Build history of the part. All positions in model axes, mm. A direction names the side the tool comes from. Round coordinates to 2 decimals unless told otherwise and drop trailing zeros. Write each loop counter-clockwise with the first axis right and the second up, starting at its lowest first coordinate (ties: lowest second). Pieces come first, ordered by that corner, then holes. Notation, with made-up numbers: (12.25, -38.75) -> (21.25, -38.75) arc R23 cw to (21.25, -11.75) -> close; hole circle Ø8 at (-16.5, 4). An arc over 180 degrees is marked (long way). Answer in a Markdown table with one row per item.
```python
from build123d import *

# Parameters (mm, degrees)
F0_W          = 203.2
F0_H          = 203.2
F1_DEPTH      = 304.8
F2_W          = 127
F2_H          = 228.6
F3_DEPTH      = 25.4
F3_DEPTH_BACK = 203.2


with BuildPart() as f1:
    # F0 (on Front) → F1 (new body)
    with BuildSketch(Plane.XZ):
        Rectangle(F0_W, F0_H)
    extrude(amount=-F1_DEPTH)

    # F2 (on face) → F3 (cut, two sides)
    with BuildSketch(Plane.XY.offset(101.6)) as f3_sk:
        with Locations((0, 152.4)):
            Rectangle(F2_W, F2_H)
    extrude(amount=F3_DEPTH, mode=Mode.SUBTRACT)
    extrude(f3_sk.sketch, amount=-F3_DEPTH_BACK, mode=Mode.SUBTRACT)


solid = f1.part
```
Q1. Which spindle directions (+Z, -Z, +X, -X, +Y, -Y) get a long thin tool onto all of the face, cutting with end or side? Do faces 5 (the flat face through (-1, 38.1, 1)), 6 (the flat face through (66, 150, -101.6)). Say none if no direction does.
A:
| item | result |
|---|---|
| face 5 | +Z, -Z |
| face 6 | -Z, +X, -X, +Y, -Y |
Q2. Wall check: line 1 (Y direction, x = 23, z = -2.5); line 2 (X direction, y = 178.5, z = 87). Give the ranges that are in metal, low to high. Write a range as [from, to].
A:
| item | result |
|---|---|
| line 1 | [0, 38.1], [266.7, 304.8] |
| line 2 | [-101.6, -63.5], [63.5, 101.6] |
Q3. Saw through at A-A on x = 19. Write the cut outline in (y, z).
A:
| item | result |
|---|---|
| outline | (0, -101.6) -> (38.1, -101.6) -> (38.1, 101.6) -> (0, 101.6) -> close; (266.7, -101.6) -> (304.8, -101.6) -> (304.8, 101.6) -> (266.7, 101.6) -> close |
Q4. Saw through at C-C on z = -58.5. Write the cut outline in (x, y), plus the area to 3 significant figures.
A:
| item | result |
|---|---|
| outline | (-101.6, 0) -> (101.6, 0) -> (101.6, 304.8) -> (-101.6, 304.8) -> close; hole (-63.5, 38.1) -> (63.5, 38.1) -> (63.5, 266.7) -> (-63.5, 266.7) -> close |
| area | 32,900 mm² |
Q5. Two-plate mould, pull along Y, no slides. Class faces 1 (the flat face through (-1, 304.8, 1)), 2 (the flat face through (-1, 0, 1)), 3 (the flat face through (66, 150, 101.6)), 4 (the flat face through (63.5, 151, 1)): released by +Y, released by -Y, zero draft, split by the parting line, or undercut.
A:
| item | result |
|---|---|
| face 1 | released by +Y |
| face 2 | released by -Y |
| face 3 | zero draft |
| face 4 | undercut |
Q6. Saw through at B-B on y = 231.5. Write the cut outline in (x, z).
A:
| item | result |
|---|---|
| outline | (-101.6, -101.6) -> (-63.5, -101.6) -> (-63.5, 101.6) -> (-101.6, 101.6) -> close; (63.5, -101.6) -> (101.6, -101.6) -> (101.6, 101.6) -> (63.5, 101.6) -> close |
Q7. Drop a flat-ended pin along its axis: P1, Ø1.5, axis at x = 54.5, z = 5, coming from the -Y side. Give the stop position or say it passes through.
A:
| item | result |
|---|---|
| P1 | y = 0 |
